Solid Edge part; units mm, degrees
sketch "Sketch1" plane through (0, 0, 0) normal (0, 0, 1) x (1, 0, 0)
  line L0 (20.8205, 8.2233) -> (88.8205, 8.2233)
  line L1 (88.8205, 8.2233) -> (88.8205, 101.2233)
  line L2 (88.8205, 101.2233) -> (20.8205, 101.2233)
  line L3 (20.8205, 101.2233) -> (20.8205, 8.2233)
extrude "Protrusion1" add sketch "Sketch1" along normal blind 2
sketch "Sketch2" plane through (54.8205, 54.7233, 0) normal (0, 0, -1) x (1, 0, 0)
  line L0 (-34, 46.5) -> (34, 46.5)
  line L1 (34, 46.5) -> (34, 42.5)
  line L2 (34, 42.5) -> (-34, 42.5)
  line L3 (-34, 42.5) -> (-34, 46.5)
extrude "Extrusionsausprägung_2" add sketch "Sketch2" along normal blind 32
sketch "Sketch3" plane through (54.8205, 12.2233, -16) normal (0, 1, 0) x (-1, 0, 0)
  line L0 (-34, 16) -> (-34, 12)
  line L1 (-34, 12) -> (-30, 12)
  line L2 (-30, 12) -> (-30, 14)
  line L3 (-30, 14) -> (-32, 14)
  line L4 (-32, 14) -> (-32, 16)
  line L5 (-32, 16) -> (-34, 16)
  line L6 (34, 12) -> (30, 12)
  line L7 (30, 12) -> (30, 14)
  line L8 (30, 14) -> (32, 14)
  line L9 (32, 14) -> (32, 16)
  line L10 (32, 16) -> (34, 16)
  line L11 (34, 16) -> (34, 12)
extrude "Extrusionsausprägung_3" add sketch "Sketch3" along normal blind 89
sketch "Sketch4" plane through (54.8205, 54.7233, 2) normal (0, 0, 1) x (-1, 0, 0)
  line L0 (34, 46.5) -> (-34, 46.5)
  line L1 (-34, 46.5) -> (-34, 42.5)
  line L2 (-34, 42.5) -> (34, 42.5)
  line L3 (34, 42.5) -> (34, 46.5)
extrude "Extrusionsausprägung_4" add sketch "Sketch4" along normal blind 10
sketch "Sketch5" plane through (54.8205, 12.2233, 7) normal (0, 1, 0) x (-1, 0, 0)
  line L0 (-22, 5) -> (-34, -5)
  line L1 (-34, -5) -> (-30, -5)
  line L2 (-30, -5) -> (-20, 3)
  line L3 (-20, 3) -> (20, 3)
  line L4 (30, -5) -> (20, 3)
  line L5 (34, -5) -> (30, -5)
  line L6 (22, 5) -> (34, -5)
  line L7 (22, 5) -> (20, 5)
  line L8 (20, 5) -> (-20, 5)
  line L9 (-22, 5) -> (-20, 5)
extrude "Protrusion2" add sketch "Sketch5" along normal up to vertex (89 mm away)
sketch "Sketch6" plane through (26.8205, 12.2233, 7) normal (0, 1, 0) x (-1, 0, 0)
  line L0 (6, 5) -> (-6, 5)
  line L1 (-6, 5) -> (6, -5)
  line L2 (6, 5) -> (6, -5)
  line L3 (-62, -5) -> (-62, 5)
  line L4 (-62, 5) -> (-50, 5)
  line L5 (-50, 5) -> (-62, -5)
extrude "Extrusionsausschnitt_1" cut sketch "Sketch6" against normal blind 15.0999
sketch "Sketch7" plane through (54.8205, 101.2233, 4) normal (0, 1, 0) x (-1, 0, 0)
  line L0 (30, -2) -> (30, -4)
  line L1 (-30, -4) -> (30, -4)
  line L2 (-30, -2) -> (-30, -4)
  line L3 (30, -2) -> (-30, -2)
extrude "Extrusionsausschnitt_2" cut sketch "Sketch7" against normal blind 88.9965
sketch "Sketch8" plane through (54.8205, 12.2233, 6) normal (0, 1, 0) x (-1, 0, 0)
  line L0 (20, 4) -> (20, 2)
  line L1 (20, 2) -> (16, 2)
  line L2 (16, 2) -> (25, -6)
  line L3 (25, -6) -> (30, -6)
  line L4 (30, -6) -> (30, -4)
  line L5 (30, -4) -> (20, 4)
  line L6 (-20, 4) -> (-20, 2)
  line L7 (-20, 2) -> (-16, 2)
  line L8 (-16, 2) -> (-25, -6)
  line L9 (-25, -6) -> (-30, -6)
  line L10 (-30, -6) -> (-30, -4)
  line L11 (-30, -4) -> (-20, 4)
extrude "Extrusionsausprägung_6" add sketch "Sketch8" along normal blind 46
sketch "Sketch9" plane through (34.8205, 35.2233, 9) normal (1, 0, 0) x (0, -1, 0)
  line L0 (-39, -1) -> (-44.5, -1)
  line L1 (-39, 0.5) -> (-44.5, -1)
  line L2 (-39, -1) -> (-39, 0.5)
extrude "Protrusion3" add sketch "Sketch9" along normal up to vertex (40 mm away)
sketch "Sketch10" plane through (20.8205, 54.7233, -15) normal (-1, 0, 0) x (0, -1, 0)
  line L0 (42.5, -17) -> (42.5, -13)
  line L1 (42.5, -13) -> (46.5, -13)
  line L2 (46.5, -13) -> (46.5, -17)
  line L3 (46.5, -17) -> (42.5, -17)
extrude "Extrusionsausschnitt_3" cut sketch "Sketch10" against normal blind 105.6963
sketch "Sketch11" plane through (54.8205, 8.2233, -8) normal (0, -1, 0) x (1, 0, 0)
  line L0 (-28, -20) -> (-28, -4)
  line L1 (28, -4) -> (-28, -4)
  line L2 (28, -20) -> (28, -4)
  line L3 (-28, -20) -> (28, -20)
extrude "Extrusionsausschnitt_4" cut sketch "Sketch11" against normal blind 79.8012
sketch "Sketch12" plane through (54.8205, 54.7233, 12) normal (0, 0, 1) x (-1, 0, 0)
  line L0 (20, 42.5) -> (20, 2.5)
  line L1 (20, 2.5) -> (-20, 2.5)
  line L2 (-20, 2.5) -> (-20, 42.5)
  line L3 (-20, 42.5) -> (20, 42.5)
  line L4 (-18, 40.5) -> (-18, 4.5)
  line L5 (-18, 4.5) -> (18, 4.5)
  line L6 (18, 4.5) -> (18, 40.5)
  line L7 (18, 40.5) -> (-18, 40.5)
extrude "Extrusionsausschnitt_5" cut sketch "Sketch12" against normal blind 0.5
sketch "Sketch13" plane through (54.8205, 12.2233, -14) normal (0, 1, 0) x (-1, 0, 0)
  line L0 (34, -18) -> (28, -18)
  line L1 (28, -18) -> (28, -14)
  line L2 (28, -14) -> (34, -14)
  line L3 (34, -14) -> (34, -18)
  line L4 (-28, -14) -> (-28, -18)
  line L5 (-28, -18) -> (-34, -18)
  line L6 (-34, -18) -> (-34, -14)
  line L7 (-34, -14) -> (-28, -14)
extrude "Protrusion4" add sketch "Sketch13" against normal blind 4
sketch "Sketch14" plane through (54.8205, 8.2233, -10) normal (0, -1, 0) x (1, 0, 0)
  circle A0 centre (-31, -19) radius 0.5
  circle A1 centre (31, -19) radius 0.5
extrude "Extrusionsausschnitt_6" cut sketch "Sketch14" against normal blind 44.3708
sketch "Sketch15" plane through (54.8205, 8.2233, -10) normal (0, -1, 0) x (1, 0, 0)
  line L0 (-28, -2) -> (-28, 3)
  line L1 (-28, 3) -> (28, 3)
  line L2 (28, 3) -> (28, -2)
  line L3 (28, -2) -> (-28, -2)
extrude "Extrusionsausschnitt_7" cut sketch "Sketch15" against normal blind 62.3591
sketch "Sketch16" plane through (31.8205, 58.2233, 5) normal (0, 1, 0) x (-1, 0, 0)
  line L0 (-7, 3) -> (-7, 0)
  line L1 (-7, 0) -> (-1, 0)
  line L2 (-1, 0) -> (-1, 3.4)
  line L3 (-1, 3.4) -> (-3, 5)
  line L4 (-3, 5) -> (-7, 5)
  line L5 (-7, 5) -> (-7, 3)
  line L6 (-39, 0) -> (-45, 0)
  line L7 (-45, 0) -> (-45, 3.4)
  line L8 (-45, 3.4) -> (-43, 5)
  line L9 (-43, 5) -> (-39, 5)
  line L10 (-39, 5) -> (-39, 0)
extrude "Cutout1" cut sketch "Sketch16" against normal up to vertex (46 mm away)
sketch "Sketch17" plane through (54.8205, 12.2269, 1) normal (0, 1, 0) x (1, 0, 0)
  line L0 (19.375, -4) -> (17.375, -4)
  line L1 (17.375, -4) -> (25, 1)
  line L2 (25, 1) -> (19.375, -4)
  line L3 (-19.375, -4) -> (-17.375, -4)
  line L4 (-17.375, -4) -> (-25, 1)
  line L5 (-25, 1) -> (-19.375, -4)
extrude "Protrusion5" add sketch "Sketch17" along normal blind 45.9956
sketch "Sketch18" plane through (54.8205, 101.2233, 4) normal (0, 1, 0) x (1, 0, 0)
  line L0 (-30, 6) -> (-30.5, 6)
  line L1 (-30.5, 7.5) -> (-30.5, 6)
  line L2 (-34, 7.5) -> (-30.5, 7.5)
  line L3 (-34, 8) -> (-34, 7.5)
  line L4 (-34, 8) -> (-30, 8)
  line L5 (-30, 6) -> (-30, 8)
  line L6 (34, 7.5) -> (30.5, 7.5)
  line L7 (30.5, 7.5) -> (30.5, 6)
  line L8 (30.5, 6) -> (30, 6)
  line L9 (30, 6) -> (30, 8)
  line L10 (30, 8) -> (34, 8)
  line L11 (34, 8) -> (34, 7.5)
extrude "Cutout2" cut sketch "Sketch18" against normal up to vertex (89 mm away)
sketch "Sketch19" plane through (54.8205, 32.2233, 12) normal (0, 0, 1) x (-1, 0, 0)
  circle A0 centre (0, 0) radius 2
  arc A1 (2.8284, 2.8284) -> (2.8284, -2.8284) centre (0, 0) cw
  line L0 (2.8284, -2.8284) -> (4.2426, -4.2426)
  arc A2 (4.2426, 4.2426) -> (4.2426, -4.2426) centre (0, 0) cw
  line L1 (2.8284, 2.8284) -> (4.2426, 4.2426)
  arc A3 (5.6569, 5.6569) -> (5.6569, -5.6569) centre (0, 0) cw
  line L2 (5.6569, -5.6569) -> (7.0711, -7.0711)
  arc A4 (7.0711, 7.0711) -> (7.0711, -7.0711) centre (0, 0) cw
  line L3 (5.6569, 5.6569) -> (7.0711, 7.0711)
  arc A5 (8.4853, 8.4853) -> (8.4853, -8.4853) centre (0, 0) cw
  line L4 (8.4853, -8.4853) -> (9.8995, -9.8995)
  arc A6 (9.8995, 9.8995) -> (9.8995, -9.8995) centre (0, 0) cw
  line L5 (8.4853, 8.4853) -> (9.8995, 9.8995)
  arc A7 (-2.8284, 2.8284) -> (-2.8284, -2.8284) centre (0, 0) ccw
  line L6 (-4.2426, -4.2426) -> (-2.8284, -2.8284)
  arc A8 (-4.2426, 4.2426) -> (-4.2426, -4.2426) centre (0, 0) ccw
  line L7 (-4.2426, 4.2426) -> (-2.8284, 2.8284)
  arc A9 (-5.6569, 5.6569) -> (-5.6569, -5.6569) centre (0, 0) ccw
  line L8 (-7.0711, -7.0711) -> (-5.6569, -5.6569)
  arc A10 (-7.0711, 7.0711) -> (-7.0711, -7.0711) centre (0, 0) ccw
  line L9 (-7.0711, 7.0711) -> (-5.6569, 5.6569)
  arc A11 (-8.4853, 8.4853) -> (-8.4853, -8.4853) centre (0, 0) ccw
  line L10 (-9.8995, -9.8995) -> (-8.4853, -8.4853)
  arc A12 (-9.8995, 9.8995) -> (-9.8995, -9.8995) centre (0, 0) ccw
  line L11 (-8.4853, 8.4853) -> (-9.8995, 9.8995)
extrude "Cutout3" cut sketch "Sketch19" against normal up to vertex (0.5 mm away)
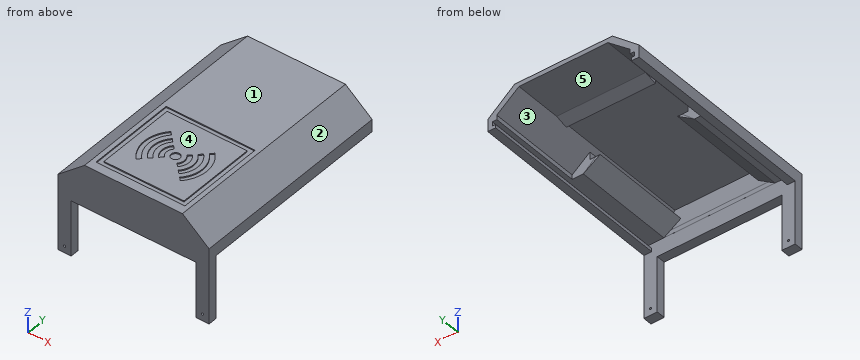
Here's how the part is built. I have some questions about the finished solid (model axes, mm). Face numbers are marked on the shaded views. A direction names the side the tool comes from. Round coordinates to 2 decimals unless told otherwise and drop trailing zeros. Loops run counter-clockwise (first coordinate to the right, second up) from the corner with the lowest first, then second, coordinate; pieces in that order, holes last.
1. Thinking about a two-plate mould opening in X: for the marked faces 1, 2 and 3, which applies, released by +X, released by -X, zero draft, split by the parting line, or undercut?
Answers:
face 1: zero draft
face 2: released by +X
face 3: undercut
2. Suppose I cut it at A-A, the plane z = -10.5. Please give me the cut outline in (x, y).
Answers:
outline: (20.82, 8.22) - (26.82, 8.22) - (26.82, 12.22) - (20.82, 12.22) - close; (82.82, 8.22) - (88.82, 8.22) - (88.82, 12.22) - (82.82, 12.22) - close
3. Will these pins go through, and if not, where does the flat tip stop? pin 1 (0.8 mm diameter, centred on x = 23.5, y = 37.5, fed in from +Z); pin 2 (2.5 mm diameter, centred on x = 29, z = 3, fed in from +Y); pin 3 (1.6 mm diameter, centred on x = 65, z = 1, fed in from +Y).
Answers:
pin 1: stops at z = 4.57
pin 2: stops at y = 58.22
pin 3: stops at y = 12.23
4. Suppose I cut it at D-D, the plane z = -6. Please give me the cut outline in (x, y), and give its area (3 significant figures).
Answers:
outline: (20.82, 8.22) - (88.82, 8.22) - (88.82, 12.22) - (20.82, 12.22) - close
area: 272 mm2
5. Suppose I cut it at C-C, the plane y = 75.5. Please give me the cut outline in (x, z), and give its area (3 significant figures).
Answers:
outline: (20.82, -3.5) - (24.32, -3.5) - (24.32, -2) - (22.82, -2) - (22.82, 0) - (24.82, 0) - (24.82, 2) - (34.82, 10) - (34.82, 8.85) - (74.82, 8.85) - (74.82, 10) - (84.82, 2) - (84.82, 0) - (86.82, 0) - (86.82, -2) - (85.32, -2) - (85.32, -3.5) - (88.82, -3.5) - (88.82, 2) - (76.82, 12) - (32.82, 12) - (20.82, 2) - close
area: 241 mm2
6. For the marked faces 4 and 5, which set-ups out of +Z, -Z, +X, -X, +Y, -Y let a thin tool reach every point of the face, with its end or its side?
Answers:
face 4: +Z, +X, -X, +Y, -Y
face 5: -Z, +Y
7. If I drill on probe 1 along Z at (x, y) = (42.5, 64); probe 2 along Y at (x, z) = (61.5, 4); probe 3 along Z at (x, y) = (70, 14), over which ranges is the centre line in solid material (lowest first)?
Answers:
probe 1: z = 10 to 12
probe 2: y = 8.22 to 12.22
probe 3: z = 10 to 11.5
